Geometry: final body of the model. Coordinates: model frame, mm. Face numbers are marked on the shaded views. Round coordinates to 2 decimals unless told otherwise and drop trailing zeros. Loops run counter-clockwise (first coordinate to the right, second up) from the corner with the lowest first, then second, coordinate; pieces in that order, holes last. Notation, with made-up numbers: M -30,88.25 L 28,88.25 A6 cw 28,94.25 Z; hole C -10,38 d2. An arc over 180 degrees is marked long. Answer as a JSON object with one key per item and string values.
```python
from build123d import *

# Parameters (mm, degrees)
BOSS_EXTRUDE1_DEPTH    = 17
M6_TAPPED_HOLE1_D      = 5
CUT_EXTRUDE1_REACH     = 27.02
SKETCH5_R              = 3.1
M3_TAPPED_HOLE1_REACH  = 28.019
M3_TAPPED_HOLE1_BORE_R = 1.25
M3_TAPPED_HOLE2_D      = 2.5
SKETCH13_R             = 1
CUT_EXTRUDE2_DEPTH     = 16.2
CUT_EXTRUDE3_START     = 3.5
CUT_EXTRUDE3_DEPTH     = 2
FILLET1_R              = 0.1


with BuildPart() as part:
    # Sketch1 → Boss-Extrude1 (new body)
    with BuildSketch(Plane(origin=(0, 0, 0), x_dir=(1, 0, 0), z_dir=(0, 1, 0))):
        with BuildLine():
            Line((-7, 8), (7, 8))
            ThreePointArc((7, 8), (8.414213562, 7.414213562), (9, 6))
            Line((9, 6), (9, -6))
            ThreePointArc((9, -6), (8.414213562, -7.414213562), (7, -8))
            Line((7, -8), (-7, -8))
            ThreePointArc((-7, -8), (-8.414213562, -7.414213562), (-9, -6))
            Line((-9, -6), (-9, 6))
            ThreePointArc((-9, 6), (-8.414213562, 7.414213562), (-7, 8))
        make_face()
    extrude(amount=BOSS_EXTRUDE1_DEPTH)

    # M6 Tapped Hole1 (through all)
    with Locations(Plane(origin=(0, 17, 0), x_dir=(1, 0, 0), z_dir=(0, 1, 0))):
        with Locations((4.5, 0)):
            Hole(M6_TAPPED_HOLE1_D / 2)

    # Sketch5 → Cut-Extrude1 (cut, up to next)
    with BuildSketch(Plane.XY.offset(8), mode=Mode.PRIVATE) as cut_extrude1_sk1:
        with Locations((-2.9, 5.1)):
            Circle(SKETCH5_R)
    cut_extrude1_tool1 = extrude(cut_extrude1_sk1.sketch, amount=-CUT_EXTRUDE1_REACH, mode=Mode.PRIVATE) & part.part
    add(cut_extrude1_tool1.solids().sort_by_distance((-2.9, 5.1, 8))[0], mode=Mode.SUBTRACT)

    # M3 Tapped Hole1 bore → M3 Tapped Hole1 (cut, up to next)
    with BuildSketch(Plane.ZY.offset(9), mode=Mode.PRIVATE) as m3_tapped_hole1_sk1:
        with Locations((0, 5.1)):
            Circle(M3_TAPPED_HOLE1_BORE_R)
    m3_tapped_hole1_tool1 = extrude(m3_tapped_hole1_sk1.sketch, amount=-M3_TAPPED_HOLE1_REACH, mode=Mode.PRIVATE) & part.part
    add(m3_tapped_hole1_tool1.solids().sort_by_distance((-9, 5.1, 0))[0], mode=Mode.SUBTRACT)

    # M3 Tapped Hole2 (through all)
    with Locations(Plane.XY.offset(8)):
        with Locations((-1, 12.9)):
            Hole(M3_TAPPED_HOLE2_D / 2)

    # Sketch13 → Cut-Extrude2 (cut)
    with BuildSketch(Plane(origin=(0, 17.880667156, -3.496925738), x_dir=(1, 0, 0), z_dir=(0, 0.9814078107791567, -0.19193412656863024))):
        with Locations(Location((4.5, 4.588382335, 0), (0, 0, 270))):
            Circle(SKETCH13_R)
    extrude(amount=-CUT_EXTRUDE2_DEPTH, mode=Mode.SUBTRACT)

    # Cut-Extrude3: read off the stored shape, not the designer's step
    # Cut-Extrude3 outline → Cut-Extrude3 (cut)
    with BuildSketch(Plane.YZ.offset(CUT_EXTRUDE3_START)):
        Polygon((17, -8), (11.8, -6.983034935), (11.8, -8), align=None)
    extrude(amount=CUT_EXTRUDE3_DEPTH, mode=Mode.SUBTRACT)

    # Fillet1
    fillet1_edges = [part.edges().sort_by_distance(p)[0] for p in [
        (8.414213562, 0, -7.414213562),
        (9, 0, 0),
        (8.414213562, 0, 7.414213562),
        (0, 0, 8),
        (-8.414213562, 0, 7.414213562),
        (-9, 0, 0),
        (-8.414213562, 0, -7.414213562),
        (6.25, 17, -8),
        (8.414213562, 17, -7.414213562),
        (9, 17, 0),
        (8.414213562, 17, 7.414213562),
        (0, 17, 8),
        (-8.414213562, 17, 7.414213562),
        (-9, 17, 0),
        (-8.414213562, 17, -7.414213562),
        (-6, 5.1, 8),
        (0, 0, -8),
        (-6, 5.1, -8),
        (-1.75, 17, -8),
    ]]
    fillet(fillet1_edges, radius=FILLET1_R)


solid = part.part
```
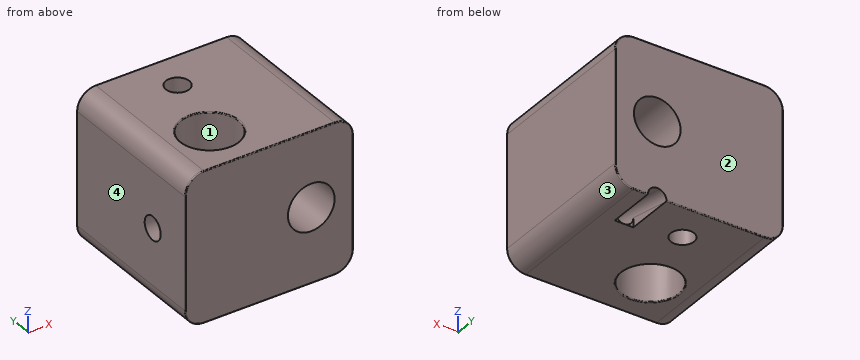
1) Cut plane C-C on z = 0. Return the cut outline in (x, y), and give its area (3 significant figures).
Geometry results:
{"outline": "M -9,0.1 A0.1 ccw -8.9,0 L 2,0 L 2,17 L -8.9,17 A0.1 ccw -9,16.9 L -9,6.35 L -5.74,6.35 A3.1 cw long -5.74,3.85 L -9,3.85 Z; M 7,0 L 8.9,0 A0.1 ccw 9,0.1 L 9,16.9 A0.1 ccw 8.9,17 L 7,17 Z; hole C -1,12.9 d2.5", "area": "178 mm2"}
2) Cut plane B-B on x = -2.9. Return the cut outline in (y, z), and give its area (3 significant figures).
Geometry results:
{"outline": "M 0,-7.9 A0.1 ccw 0.1,-8 L 1.9,-8 A0.1 ccw 2,-7.9 L 2,7.9 A0.1 ccw 1.9,8 L 0.1,8 A0.1 ccw 0,7.9 Z; M 8.2,-7.9 A0.1 ccw 8.3,-8 L 16.9,-8 A0.1 ccw 17,-7.9 L 17,7.9 A0.1 ccw 16.9,8 L 8.3,8 A0.1 ccw 8.2,7.9 Z", "area": "173 mm2"}
3) Line query: probe 1 along Y at (x, z) = (-2.9, -2); probe 2 along X at (y, z) = (12.25, -7.5); probe 3 along Z at (x, y) = (-7.1, 5.1). Output: solid intervals per line, ascending.
Geometry results:
{"probe 1": "0 to 2, 8.2 to 17", "probe 2": "-8.32 to -2.07, 0.07 to 3.5, 5.5 to 8.32", "probe 3": "-8 to -1.25, 1.25 to 8"}
4) First-contact query: pin 1 (0.8 mm diameter, centred on y = 13.5, z = -7.5, fed in from -X). Flat tip, straight axial feed; report the tip coordinate or a pass-through.
Geometry results:
{"pin 1": "x = -8.67"}
5) Cut plane A-A on z = 2. Return the cut outline in (x, y).
Geometry results:
{"outline": "M -9,0.1 A0.1 ccw -8.9,0 L 3,0 L 3,17 L -8.9,17 A0.1 ccw -9,16.9 Z; M 6,0 L 8.9,0 A0.1 ccw 9,0.1 L 9,16.9 A0.1 ccw 8.9,17 L 6,17 Z; hole C -2.9,5.1 d6.2; hole C -1,12.9 d2.5"}
6) Pull-direction query (X, two-part tool) for the marked faces 1, 2, 3 and 4; classes: +X half, -X half, draft (parallel to the pull), parting line (faces both ways), or undercut.
Geometry results:
{"face 1": "undercut", "face 2": "draft", "face 3": "+X half", "face 4": "-X half"}
7) Cut plane D-D on z = -2.75. Return the cut outline in (x, y).
Geometry results:
{"outline": "M -9,0.1 A0.1 ccw -8.9,0 L 8.9,0 A0.1 ccw 9,0.1 L 9,16.9 A0.1 ccw 8.9,17 L -8.9,17 A0.1 ccw -9,16.9 Z; hole C -2.9,5.1 d6.2; hole C -1,12.9 d2.5"}
